Design review of the part built by this model. Coordinates are the model's own, in mm. Coordinates: 2 decimals unless noted, no trailing zeros. Order: outer loops, then holes, each group sorted by start corner. A loop starts at its lowest first (then second) coordinate and runs counter-clockwise, first axis right, second up. Notation, with made-up numbers: (73.5, 85.5) -> (106.5, 85.5) arc R27 cw to (106.5, 112.5) -> close; hole circle Ø6 at (19, 47). An arc over 180 degrees is marked (long way). Use a Markdown table: item, result. Add a question column.
Q1. Add section B-B (z = -524.5). State the section outline as (x, y) points.
Q2. Add section C-C (x = 894.5). State the section outline as (y, z) points, then the cut area to 3 significant figures.
Q3. Insertion check: pin 1 (6 mm diameter, centred on y = 7.5, z = -633.5, fed in from -X); pin 2 (10 mm diameter, centred on y = 13, z = -29, fed in from +X); pin 3 (6 mm diameter, centred on y = 6, z = -244.5, fed in from +X). Each pin has a flat end and moves straight along its axis. Give the tip position at first contact, or say it passes through.
Q4. Add section D-D (z = -5). State the section outline as (x, y) points.
Q5. Add section A-A (z = -681.5). State the section outline as (x, y) points, then the cut area to 3 significant figures.
Q6. Wall thickness on probe 1 along X at (y, z) = (11.75, -607.5); probe 2 along X at (y, z) = (10.25, -574); probe 3 along Z at (x, y) = (1480.5, 18.5): over which ranges is each line inside the solid? List them lowest first.
from build123d import *

# Parameters (mm, degrees)
SKETCH1_W           = 200
SKETCH1_H           = 200
SKETCH1_W_2         = 20
SKETCH1_H_2         = 500
SKETCH1_H_3         = 50
SKETCH1_H_4         = 100
BOSS_EXTRUDE1_DEPTH = 20


with BuildPart() as part:
    # Sketch1 → Boss-Extrude1 (new body)
    with BuildSketch(Plane(origin=(0, 0, 0), x_dir=(1, 0, 0), z_dir=(0, 1, 0))):
        Rectangle(SKETCH1_W, SKETCH1_H)
        with Locations((0, 350)):
            Rectangle(SKETCH1_W_2, SKETCH1_H_2)
        with BuildLine():
            Line((-10, 600), (10, 600))
            ThreePointArc((10, 600), (200, 790), (390, 600))
            Line((390, 600), (410, 600))
            ThreePointArc((410, 600), (200, 810), (-10, 600))
        make_face()
        with Locations((400, 575)):
            Rectangle(SKETCH1_W_2, SKETCH1_H_3)
        with BuildLine():
            Line((390, 550), (410, 550))
            ThreePointArc((410, 550), (500, 460), (590, 550))
            Line((590, 550), (610, 550))
            ThreePointArc((610, 550), (500, 440), (390, 550))
        make_face()
        with Locations((600, 575)):
            Rectangle(SKETCH1_W_2, SKETCH1_H_3)
        with Locations((600, 650)):
            Rectangle(SKETCH1_W_2, SKETCH1_H_4)
        Polygon((590, 720), (590, 700), (610, 700), (1590, 700), (1590, 720), align=None)
        Polygon((1590, 720), (1590, 700), (1590, 610), (1790, 610), (1790, 810), (1590, 810), align=None)
    extrude(amount=BOSS_EXTRUDE1_DEPTH)


solid = part.part
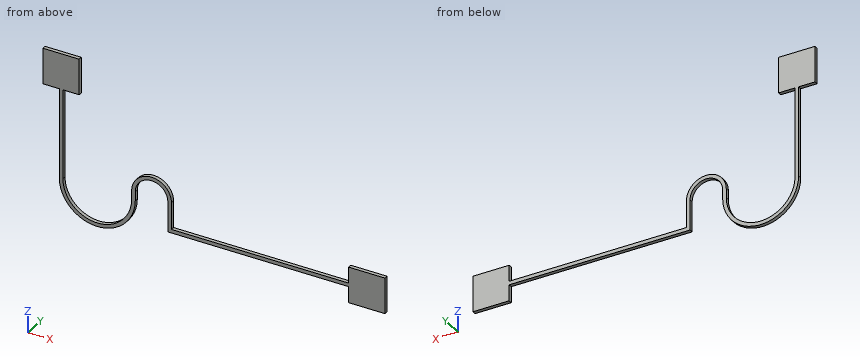
Established:
| question | item | result |
|---|---|---|
| 1 | outline | (-10, 0) -> (10, 0) -> (10, 20) -> (-10, 20) -> close; (393, 0) -> (413.69, 0) -> (413.69, 20) -> (393, 20) -> close; (586.31, 0) -> (607, 0) -> (607, 20) -> (586.31, 20) -> close |
| 2 | outline | (0, -720) -> (20, -720) -> (20, -700) -> (0, -700) -> close |
| 2 | area | 400 mm^2 |
| 3 | pin 1 | x = -7.77 |
| 3 | pin 2 | x = 100 |
| 3 | pin 3 | x = 10 |
| 4 | outline | (-100, 0) -> (100, 0) -> (100, 20) -> (-100, 20) -> close |
| 5 | outline | (6.46, 0) -> (28.37, 0) -> (28.37, 20) -> (6.46, 20) -> close; (371.63, 0) -> (393.54, 0) -> (393.54, 20) -> (371.63, 20) -> close; (590, 0) -> (610, 0) -> (610, 20) -> (590, 20) -> close; (1590, 0) -> (1790, 0) -> (1790, 20) -> (1590, 20) -> close |
| 5 | area | 5,280 mm^2 |
| 6 | probe 1 | -9.87 to 10.15, 389.85 to 409.87, 590 to 610 |
| 6 | probe 2 | -10 to 10, 390 to 410, 590 to 610 |
| 6 | probe 3 | -720 to -700 |
